from build123d import *

# Parameters (mm, degrees)
BOSS_EXTRUDE2_DEPTH = 2.5
SKETCH4_R           = 0.99
CUT_EXTRUDE2_DEPTH  = 64.988660757
SKETCH6_R           = 0.99
BOSS_EXTRUDE4_DEPTH = 2.8
SKETCH7_W           = 2.01987101
SKETCH7_H           = 0.78494751
BOSS_EXTRUDE5_DEPTH = 2.5


with BuildPart() as part:
    # Sketch3 → Boss-Extrude2 (new body)
    with BuildSketch(Plane(origin=(0, 0, 0), x_dir=(0, 0, -1), z_dir=(1, 0, 0))):
        with BuildLine():
            Line((-54.67077374, 30.968825597), (-55.447230875, 28.071048118))
            ThreePointArc((-55.447230875, 28.071048118), (-53.67077374, 25.652507451), (-51.894316605, 28.071048118))
            Line((-51.894316605, 28.071048118), (-52.67077374, 30.968825597))
            ThreePointArc((-52.67077374, 30.968825597), (-53.67077374, 31.692969852), (-54.67077374, 30.968825597))
        make_face()
    extrude(amount=BOSS_EXTRUDE2_DEPTH)

    # Sketch4 → Cut-Extrude2 (cut, through all)
    with BuildSketch(Plane(origin=(2.5, 0, 0), x_dir=(0, 0, -1), z_dir=(1, 0, 0))):
        with Locations((-53.67077374, 27.514195996)):
            Circle(SKETCH4_R)
    extrude(amount=-CUT_EXTRUDE2_DEPTH, mode=Mode.SUBTRACT)

    # Sketch6 → Boss-Extrude4 (add)
    with BuildSketch(Plane(origin=(2.5, 0, 0), x_dir=(0, 0, -1), z_dir=(1, 0, 0))):
        with Locations((-53.67077374, 30.640427563)):
            Circle(SKETCH6_R)
    extrude(amount=BOSS_EXTRUDE4_DEPTH)

    # Sketch7 → Boss-Extrude5 (add)
    with BuildSketch(Plane(origin=(2.5, 0, 0), x_dir=(0, 0, -1), z_dir=(1, 0, 0))):
        with Locations((-53.657499813, 28.408869671)):
            Rectangle(SKETCH7_W, SKETCH7_H)
    extrude(amount=-BOSS_EXTRUDE5_DEPTH)


solid = part.part
Source: CAD feature listing. Evaluate the final solid. Frame: model axes, mm. A direction names the side the tool comes from. Coordinates: 2 decimals unless noted, no trailing zeros. Loops run counter-clockwise (first coordinate to the right, second up) from the corner with the lowest first, then second, coordinate; pieces in that order, holes last. Notation, with made-up numbers: (-9, 29) -> (48, 29) arc R15 ccw to (48, 35) -> close; hole circle Ø7 at (77.5, 6). An arc over 180 degrees is marked (long way). Answer in a Markdown table with one row per item. Add a question column.
Q1. Section D-D on z = 53.9. Return the cut outline in (x, y), and give its area (3 significant figures).
Q2. Contact query for flat-ended pins moving along their axis: pin 1 Ø1.5 at (x, y) = (3.5, 30.5) entering from +Z; pin 2 Ø1.5 at (x, y) = (0.5, 30.5) entering from -Z. Output: stop coordinate, or through.
Q3. Section A-A on x = 1. Return the cut outline in (y, z), and give its area (3 significant figures).
Q4. Ray query, line 1 along Y through (x, z) = (1.2, 54.4); line 2 along X through (y, z) = (28.75, 54.8); line 3 along Z through (x, y) = (0.85, 26.75). Return the intervals inside material, ascending.
Q5. Reachability of faces 4 (the face through (5.3, 31, 54)), 5 (the face through (3.88, 31.31, 54.4)), 6 (the face through (1, 28.016, 54)) from +Z, -Z, +X, -X, +Y, -Y: full face, straight path, thin tool, end or side. Return the list, or none.
Q6. Section C-C on y = 30.5. Return the cut outline in (x, z).
Q7. Pull-direction query (Z, two-part tool) for faces 1 (the face through (0, 29, 54)), 2 (the face through (1.232, 25.653, 53.72)), 3 (the face through (1.268, 26.525, 53.7)); classes: pulls with the +Z half, pulls with the -Z half, needs draft (parallel to the pull), parting line crosses it, or undercut.
Q8. Section B-B on z = 53.15. Return the cut outline in (x, y).
Computed values:
| question | item | result |
|---|---|---|
| 1 | outline | (0, 25.67) -> (2.5, 25.67) -> (2.5, 26.55) -> (0, 26.55) -> close; (0, 28.02) -> (2.5, 28.02) -> (2.5, 29.68) -> (5.3, 29.68) -> (5.3, 31.6) -> (2.5, 31.6) -> (2.5, 31.67) -> (0, 31.67) -> close |
| 1 | area | 16.7 mm^2 |
| 2 | pin 1 | stops at z = 54.66 |
| 2 | pin 2 | stops at z = 52.34 |
| 3 | outline | (28.07, 51.89) -> (30.97, 52.67) arc R1.05 ccw to (30.97, 54.67) -> (28.07, 55.45) arc R1.86 ccw (long way) to start; hole (28.02, 52.82) -> (28.02, 54.52) arc R0.99 ccw (long way) to start |
| 3 | area | 14.1 mm^2 |
| 4 | line 1 | y = 25.8 to 26.84, 28.02 to 31.4 |
| 4 | line 2 | x = 0 to 2.5 |
| 4 | line 3 | z = 51.97 to 53.04, 54.3 to 55.37 |
| 5 | face 4 | +Z, -Z, +X, +Y, -Y |
| 5 | face 5 | +X |
| 5 | face 6 | +X, -X |
| 6 | outline | (0, 52.55) -> (2.5, 52.55) -> (2.5, 52.69) -> (5.3, 52.69) -> (5.3, 54.65) -> (2.5, 54.65) -> (2.5, 54.8) -> (0, 54.8) -> close |
| 7 | face 1 | needs draft |
| 7 | face 2 | parting line crosses it |
| 7 | face 3 | undercut |
| 8 | outline | (0, 25.73) -> (2.5, 25.73) -> (2.5, 26.67) -> (0, 26.67) -> close; (0, 28.02) -> (2.5, 28.02) -> (2.5, 29.8) -> (5.3, 29.8) -> (5.3, 31.48) -> (2.5, 31.48) -> (2.5, 31.56) -> (0, 31.56) -> close |
